Model file for the job. Use its own axes, mm. Give positions to 0.01 mm unless a question says otherwise; leave off trailing zeros. Loops run counter-clockwise (first coordinate to the right, second up) from the corner with the lowest first, then second, coordinate; pieces in that order, holes last. Notation, with made-up numbers: (45, 2) -> (54, 2) arc R16 ccw to (54, 19) -> close; hole circle Ø3 at (-33, -32.5). An arc over 180 degrees is marked (long way). Use CSV: the item, a comma, the result in double quotes. Start each with the question number.
(1) Cut at A-A on z = 516.5. Write the cut outline in (x, y).
(2) Flat gauge pins, fed straight in: pin 1 (1.5 mm diameter, centred on y = 43.5, z = 676, fed in from +X); pin 2 (6 mm diameter, centred on x = 121, z = 251, fed in from +Y); pin 3 (3 mm diameter, centred on x = 270, z = 433, fed in from +Y) (3 decimals). Where does each tip first touch, or does it go through?
(3) Drill centre lines: probe 1 along Y at (x, z) = (269.5, 393.5) (3 decimals); probe 2 along Y at (x, z) = (281.5, 512) (3 decimals). Where is each one in solid material? Low to high.
(4) Cut at B-B on y = 13. Write the cut outline in (x, z), then the cut area to 3 significant figures.
from build123d import *

# Parameters (mm, degrees)
BOSS_EXTRUDE1_DEPTH = 690
SKETCH3_W           = 30
SKETCH3_H           = 20
SKETCH3_H_2         = 30
CUT_EXTRUDE2_DEPTH  = 51


with BuildPart() as part:
    # Sketch1 → Boss-Extrude1 (new body)
    with BuildSketch(Plane.XY):
        Polygon((0, 5), (0, 0), (300, 45), (300, 50), align=None)
    extrude(amount=BOSS_EXTRUDE1_DEPTH)

    # Sketch3 → Cut-Extrude2 (cut, through all)
    with BuildSketch(Plane(origin=(0, 0, 0), x_dir=(1, 0, 0), z_dir=(0, 1, 0))):
        with Locations((285, -680)):
            Rectangle(SKETCH3_W, SKETCH3_H)
        with Locations((285, -15)):
            Rectangle(SKETCH3_W, SKETCH3_H_2)
    extrude(amount=CUT_EXTRUDE2_DEPTH, mode=Mode.SUBTRACT)


solid = part.part
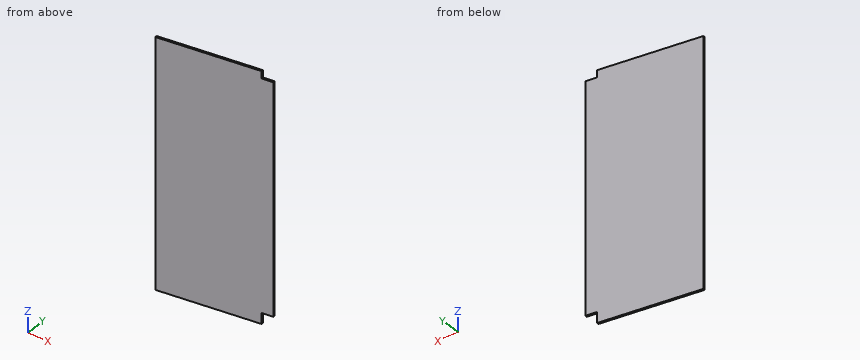
Check result:
1,outline,"(0, 0) -> (300, 45) -> (300, 50) -> (0, 5) -> close"
2,pin 1,"x = 270"
2,pin 2,"y = 23.6"
2,pin 3,"y = 45.725"
3,probe 1,"40.425 to 45.425"
3,probe 2,"42.225 to 47.225"
4,outline,"(53.33, 0) -> (86.67, 0) -> (86.67, 690) -> (53.33, 690) -> close"
4,area,"23,000 mm²"
